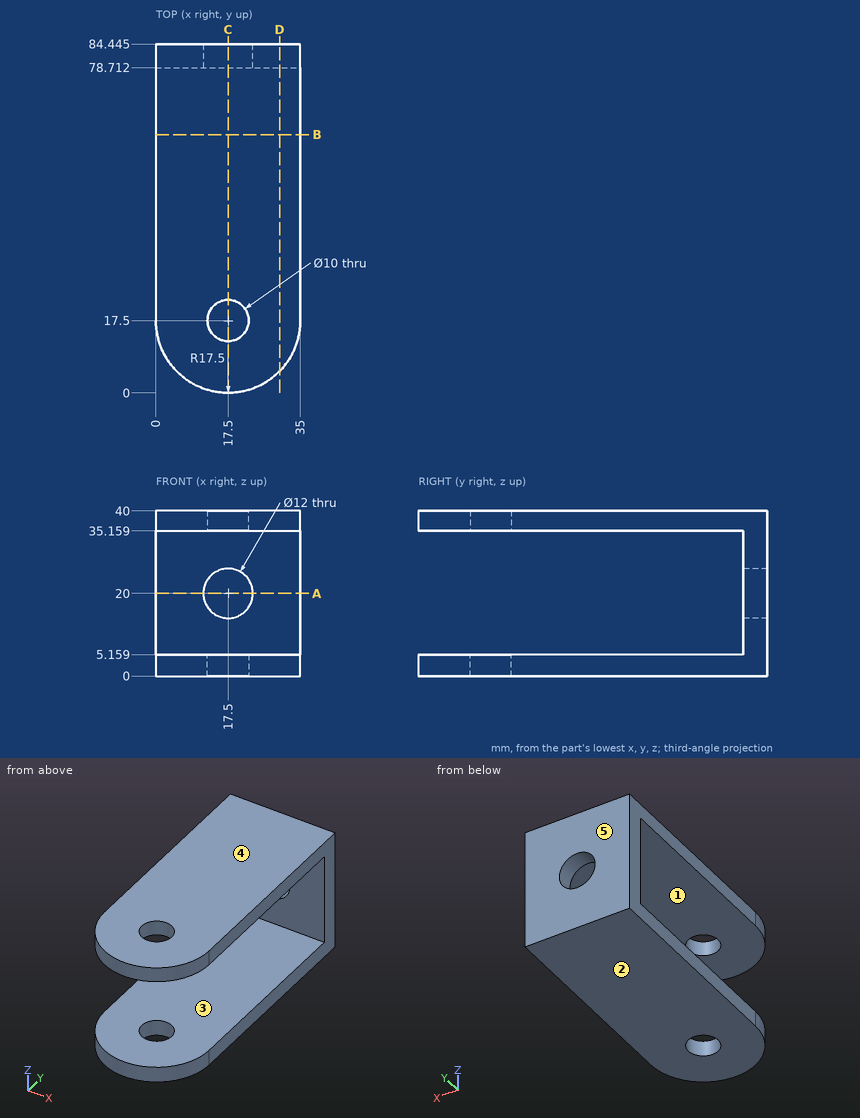
Geometry: see drawing. Coordinates: mm, zero at the bounding-box minimum. A direction names the side the tool comes from. Coordinates: 2 decimals unless noted, no trailing zeros. Loops run counter-clockwise (first coordinate to the right, second up) from the corner with the lowest first, then second, coordinate; pieces in that order, holes last.
(1) Section C-C on x = 17.5. Return the cut outline in (y, z) (1 decimal).
(2) Section D-D on x = 30. Return the cut outline in (y, z) (1 decimal).
(3) Set-up query: the marked faces 1 and 2. Return all of +Z, -Z, +X, -X, +Y, -Y with unobstructed straight access to the full face (end or side cutting, diameter ignored); none if empty.
(4) Section A-A on z = 20. Return the cut outline in (x, y) (1 decimal), then the cut area to 3 significant figures.
(5) Pull-direction query (Z, two-part tool) for the marked faces 3, 4 and 5; classes: released by +Z, released by -Z, zero draft, split by the parting line, or undercut.
(6) Material intervals for probe 1 along X at (y, z) = (17.5, 37.1); probe 2 along Z at (x, y) = (20, 22); probe 3 along Z at (x, y) = (17.5, 81.75), sorted ascending.
(7) Section B-B on y = 62.5. Return the cut outline in (x, z).
(8) First-contact query: pin 1 Ø1 at (x, y) = (15, 18) entering from -Z; pin 2 Ø9 at (x, z) = (9, 21.5) entering from -Y; pin 3 Ø4 at (x, y) = (12, 59) entering from -Z. Flat tips, straight axial feed; report the tip coordinate or a pass-through.
Data:
1. outline: (0, 0) - (12.5, 0) - (12.5, 5.2) - (0, 5.2) - close; (0, 35.2) - (12.5, 35.2) - (12.5, 40) - (0, 40) - close; (22.5, 0) - (84.4, 0) - (84.4, 14) - (78.7, 14) - (78.7, 5.2) - (22.5, 5.2) - close; (22.5, 35.2) - (78.7, 35.2) - (78.7, 26) - (84.4, 26) - (84.4, 40) - (22.5, 40) - close
2. outline: (5.3, 0) - (84.4, 0) - (84.4, 40) - (5.3, 40) - (5.3, 35.2) - (78.7, 35.2) - (78.7, 5.2) - (5.3, 5.2) - close
3. face 1: +X, -X, -Y
3. face 2: -Z, +X, -X, +Y, -Y
4. outline: (0, 78.7) - (11.5, 78.7) - (11.5, 84.4) - (0, 84.4) - close; (23.5, 78.7) - (35, 78.7) - (35, 84.4) - (23.5, 84.4) - close
4. area: 132 mm2
5. face 3: undercut
5. face 4: released by +Z
5. face 5: zero draft
6. probe 1: x = 0 to 12.5, 22.5 to 35
6. probe 2: z = 0 to 5.16, 35.16 to 40
6. probe 3: z = 0 to 14, 26 to 40
7. outline: (0, 0) - (35, 0) - (35, 5.16) - (0, 5.16) - close; (0, 35.16) - (35, 35.16) - (35, 40) - (0, 40) - close
8. pin 1: passes through
8. pin 2: stops at y = 78.71
8. pin 3: stops at z = 0
